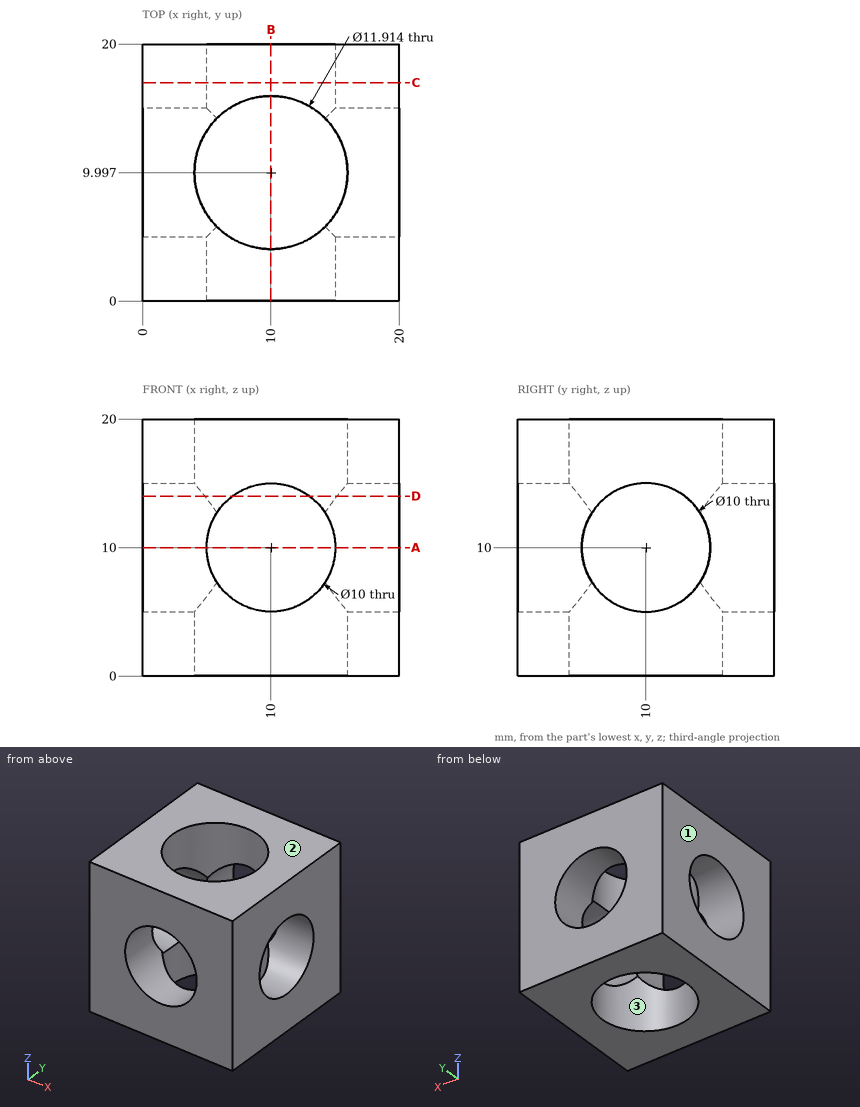
Study the drawing (mm; zero at the part's minimum x, y, z) and answer. Give positions to 0.01 mm unless a question says otherwise; leave off trailing zeros. Loops run counter-clockwise (first coordinate to the right, second up) from the corner with the lowest first, then second, coordinate; pieces in that order, holes last. Notation, with made-up numbers: (55.25, 62.5) - (85.25, 62.5) arc R25 cw to (85.25, 75.5) - close; hole circle Ø2 at (-11.75, -27.75). An arc over 180 degrees is marked (long way). Answer as CSV lines item,"result". Start each with the question number.
1) This flat-tipped pin is pushed along its axis until it touches: pin 1 Ø6 at (x, z) = (10, 10) entering from -Y. Where does it stop, or does it pass through?
2) Straight lines are drawn through the part: L1, parallel to Z at x = 10, y = 3.5; L2, parallel to X at y = 4.75, z = 9.75; L3, parallel to X at y = 14.5, z = 16.75. For each, find the intervals that lie inside material, in ascending order. Write a range as from..to.
3) Find section B-B (x = 10). Write down the section's boundary in (y, z) (1 decimal).
4) Find section A-A (z = 10). Write down the section's boundary in (x, y).
5) Find section D-D (z = 14). State how many separate pieces and enclosed holes the cut face has, then the cut area to 3 significant figures.
6) Find section C-C (y = 17). Write down the section's boundary in (x, z).
7) Determine the mould class of the marked faces 1, 2 and 3 for opening direction X: released by +X, released by -X, zero draft, split by the parting line, or undercut.
Findings below:
1,pin 1,"through"
2,L1,"0..5, 15..20"
2,L2,"0..5.01, 14.99..20"
2,L3,"0..6.1, 13.9..20"
3,outline,"(0, 0) - (4, 0) - (4, 5) - (0, 5) - close; (0, 15) - (4, 15) - (4, 20) - (0, 20) - close; (16, 0) - (20, 0) - (20, 5) - (16, 5) - close; (16, 15) - (20, 15) - (20, 20) - (16, 20) - close"
4,outline,"(0, 0) - (5, 0) - (5, 5) - (0, 5) - close; (0, 15) - (5, 15) - (5, 20) - (0, 20) - close; (15, 0) - (20, 0) - (20, 5) - (15, 5) - close; (15, 15) - (20, 15) - (20, 20) - (15, 20) - close"
5,separate pieces,"4"
5,enclosed holes,"0"
5,area,"185 mm^2"
6,outline,"(0, 0) - (20, 0) - (20, 20) - (0, 20) - close; hole circle Ø10 at (10, 10)"
7,face 1,"released by -X"
7,face 2,"zero draft"
7,face 3,"undercut"
